Model file for the job. Use its own axes, mm. Face numbers are marked on the shaded views. A direction names the side the tool comes from. Coordinates: 2 decimals unless noted, no trailing zeros. Loops run counter-clockwise (first coordinate to the right, second up) from the corner with the lowest first, then second, coordinate; pieces in that order, holes last.
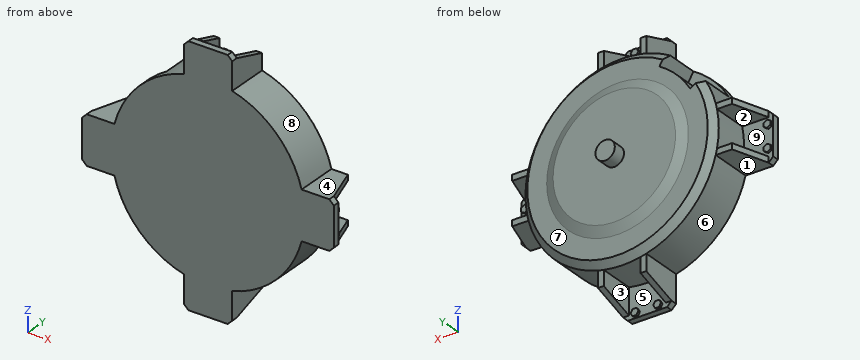
from build123d import *

# Parameters (mm, degrees)
SKETCH1_R                    = 150
BOSS_EXTRUDE1_DEPTH          = 75
CHAMFER1_SIZE                = 10
BOSS_EXTRUDE2_DEPTH          = 10
CHAMFER2_SIZE                = 7
BOSS_EXTRUDE3_DEPTH          = 9
BOSS_EXTRUDE4_DEPTH          = 3.5
CIRPATTERN1_COUNT            = 4
CIRPATTERN1_COPY_1_DEPTH     = 9
CIRPATTERN1_COPY_2_DEPTH     = 9
CIRPATTERN1_COPY_3_DEPTH     = 9
CIRPATTERN1_COPY_4_DEPTH     = 3.5
CIRPATTERN1_COPY_5_DEPTH     = 3.5
CIRPATTERN1_COPY_6_DEPTH     = 3.5
CHAMFER2_OF_CIRPATTERN1_SIZE = 7
CUT_EXTRUDE1_START           = -60
CUT_EXTRUDE1_DEPTH           = 60
SKETCH7_R                    = 110
SKETCH8_R                    = 95
SKETCH9_R                    = 15
BOSS_EXTRUDE5_DEPTH          = 20


with BuildPart() as part:
    # Sketch1 → Boss-Extrude1 (new body)
    with BuildSketch(Plane(origin=(0, 0, 0), x_dir=(1, 0, 0), z_dir=(0, 1, 0))):
        with Locations(Location((0, 0, 0), (0, 0, 270))):
            Circle(SKETCH1_R)
    extrude(amount=BOSS_EXTRUDE1_DEPTH)

    # Chamfer1
    chamfer1_edges = [part.edges().sort_by_distance(p)[0] for p in [
        (0, 75, -150),
    ]]
    chamfer(chamfer1_edges, length=CHAMFER1_SIZE)

    # Sketch2 → Boss-Extrude2 (add)
    with BuildSketch(Plane(origin=(0, 0, 0), x_dir=(-1, 0, 0), z_dir=(0, -1, 0))):
        with BuildLine():
            Line((145.236875483, 37.5), (195.236875483, 37.5))
            Line((195.236875483, 37.5), (195.236875483, -37.5))
            Line((195.236875483, -37.5), (145.236875483, -37.5))
            ThreePointArc((145.236875483, -37.5), (150, 0), (145.236875483, 37.5))
        make_face()
    boss_extrude2 = extrude(amount=-BOSS_EXTRUDE2_DEPTH)

    # Chamfer2
    chamfer2_edges = [part.edges().sort_by_distance(p)[0] for p in [
        (-195.236875483, 5, -37.5),
        (-195.236875483, 5, 37.5),
    ]]
    chamfer(chamfer2_edges, length=CHAMFER2_SIZE)

    # Sketch3 → Boss-Extrude3 (add)
    with BuildSketch(Plane.XY.offset(37.5)):
        Polygon((-145.236875483, 10), (-145.236875483, 65), (-170.556875483, 65), (-188.236875483, 10), align=None)
    boss_extrude3 = extrude(amount=-BOSS_EXTRUDE3_DEPTH)

    # Sketch4 → Boss-Extrude4 (add)
    with BuildSketch(Plane(origin=(0, 10, 0), x_dir=(1, 0, 0), z_dir=(0, 1, 0))):
        Polygon((-188.236875483, -23.54), (-183.04072306, -20.54), (-183.04072306, -14.54), (-188.236875483, -11.54), (-193.433027905, -14.54), (-193.433027905, -20.54), align=None)
    boss_extrude4 = extrude(amount=BOSS_EXTRUDE4_DEPTH)

    # Mirror1: Boss-Extrude3, Boss-Extrude4 across plane
    add(boss_extrude3.mirror(Plane.XY))
    add(boss_extrude4.mirror(Plane.XY))

    # CirPattern1: Boss-Extrude2, Boss-Extrude3, Boss-Extrude4 ×4 about axis
    cirpattern1_axis = Axis((0, 0, 0), (0, 1, 0))
    add([boss_extrude2.rotate(cirpattern1_axis, i * 360 / CIRPATTERN1_COUNT) for i in range(1, CIRPATTERN1_COUNT)])
    add([boss_extrude3.rotate(cirpattern1_axis, i * 360 / CIRPATTERN1_COUNT) for i in range(1, CIRPATTERN1_COUNT)])
    add([boss_extrude4.rotate(cirpattern1_axis, i * 360 / CIRPATTERN1_COUNT) for i in range(1, CIRPATTERN1_COUNT)])

    # CirPattern1 copy 1 sketch → CirPattern1 copy 1 (add)
    with BuildSketch(Plane(origin=(-37.5, 0, 0), x_dir=(0, 0, -1), z_dir=(-1, 0, 0))):
        Polygon((-145.236875483, -10), (-145.236875483, -65), (-170.556875483, -65), (-188.236875483, -10), align=None)
    extrude(amount=-CIRPATTERN1_COPY_1_DEPTH)

    # CirPattern1 copy 2 sketch → CirPattern1 copy 2 (add)
    with BuildSketch(Plane(origin=(0, 0, 37.5), x_dir=(-1, 0, 0), z_dir=(0, 0, 1))):
        Polygon((-145.236875483, -10), (-145.236875483, -65), (-170.556875483, -65), (-188.236875483, -10), align=None)
    extrude(amount=-CIRPATTERN1_COPY_2_DEPTH)

    # CirPattern1 copy 3 sketch → CirPattern1 copy 3 (add)
    with BuildSketch(Plane(origin=(37.5, 0, 0), x_dir=(0, 0, 1), z_dir=(1, 0, 0))):
        Polygon((-145.236875483, -10), (-145.236875483, -65), (-170.556875483, -65), (-188.236875483, -10), align=None)
    extrude(amount=-CIRPATTERN1_COPY_3_DEPTH)

    # CirPattern1 copy 4 sketch → CirPattern1 copy 4 (add)
    with BuildSketch(Plane(origin=(0, 10, 0), x_dir=(0, 0, -1), z_dir=(0, 1, 0))):
        Polygon((-188.236875483, 23.54), (-183.04072306, 20.54), (-183.04072306, 14.54), (-188.236875483, 11.54), (-193.433027905, 14.54), (-193.433027905, 20.54), align=None)
    extrude(amount=CIRPATTERN1_COPY_4_DEPTH)

    # CirPattern1 copy 5 sketch → CirPattern1 copy 5 (add)
    with BuildSketch(Plane(origin=(0, 10, 0), x_dir=(-1, 0, 0), z_dir=(0, 1, 0))):
        Polygon((-188.236875483, 23.54), (-183.04072306, 20.54), (-183.04072306, 14.54), (-188.236875483, 11.54), (-193.433027905, 14.54), (-193.433027905, 20.54), align=None)
    extrude(amount=CIRPATTERN1_COPY_5_DEPTH)

    # CirPattern1 copy 6 sketch → CirPattern1 copy 6 (add)
    with BuildSketch(Plane.ZX.offset(10)):
        Polygon((-188.236875483, 23.54), (-183.04072306, 20.54), (-183.04072306, 14.54), (-188.236875483, 11.54), (-193.433027905, 14.54), (-193.433027905, 20.54), align=None)
    extrude(amount=CIRPATTERN1_COPY_6_DEPTH)

    # Chamfer2 of CirPattern1
    chamfer2_of_cirpattern1_edges = [part.edges().sort_by_distance(p)[0] for p in [
        (-37.5, 5, 195.236875483),
        (37.5, 5, 195.236875483),
        (195.236875483, 5, 37.5),
        (195.236875483, 5, -37.5),
        (37.5, 5, -195.236875483),
        (-37.5, 5, -195.236875483),
    ]]
    chamfer(chamfer2_of_cirpattern1_edges, length=CHAMFER2_OF_CIRPATTERN1_SIZE)

    # Sketch6 → Cut-Extrude1 (cut)
    with BuildSketch(Plane(origin=(0, 75, 0), x_dir=(1, 0, 0), z_dir=(0, 1, 0)).offset(CUT_EXTRUDE1_START)):
        with BuildLine():
            Line((-112.583302492, -65), (-129.903810568, -75))
            ThreePointArc((-129.903810568, -75), (-106.066017178, -106.066017178), (-75, -129.903810568))
            Line((-75, -129.903810568), (-65, -112.583302492))
            ThreePointArc((-65, -112.583302492), (-91.923881554, -91.923881554), (-112.583302492, -65))
        make_face()
    extrude(amount=CUT_EXTRUDE1_DEPTH, mode=Mode.SUBTRACT)

    # Sketch7 → Loft1 section 0
    with BuildSketch(Plane(origin=(0, 75, 0), x_dir=(1, 0, 0), z_dir=(0, 1, 0))):
        Circle(SKETCH7_R)
    # Sketch8 → Loft1 section 1
    with BuildSketch(Plane(origin=(0, 82, 0), x_dir=(1, 0, 0), z_dir=(0, 1, 0))):
        Circle(SKETCH8_R)
    loft()

    # Sketch9 → Boss-Extrude5 (add)
    with BuildSketch(Plane(origin=(0, 82, 0), x_dir=(1, 0, 0), z_dir=(0, 1, 0))):
        with Locations(Location((0, 0, 0), (0, 0, 270))):
            Circle(SKETCH9_R)
    extrude(amount=BOSS_EXTRUDE5_DEPTH)


solid = part.part
Q1. Flat gauge pins, fed straight in: P1, Ø10, axis at x = 117.5, y = 29, coming from the -Z side; P2, Ø12, axis at x = 94.5, y = 62, coming from the +Z side; P3, Ø1.5, axis at x = -12, z = 133.5, coming from the +Y side. Where does each tip first touch, or does it go through?
Answers:
P1: stops at z = -99.22
P2: stops at z = 121.11
P3: stops at y = 75
Q2. Slice it at A-A (x = -157). List the corners of the cut face in (y, z).
Answers:
outline: (0, -37.5) - (65, -37.5) - (65, -28.5) - (10, -28.5) - (10, 28.5) - (65, 28.5) - (65, 37.5) - (0, 37.5) - close
Q3. Drill centre lines: line 1 (X direction, y = 47, z = -172.5); line 2 (X direction, y = 6.5, z = 149). Where is each one in solid material? Low to high.
Answers:
line 1: x = -37.5 to -28.5, 28.5 to 37.5
line 2: x = -37.5 to 37.5
Q4. Which spindle directions (+Z, -Z, +X, -X, +Y, -Y) get a long thin tool onto all of the face, cutting with end or side? Do the marked faces 1, 2, 3, 4 and 5. Say none if no direction does.
Answers:
face 1: -Z, -X, +Y, -Y
face 2: -X, +Y
face 3: -Z, +Y
face 4: +Z, +X, +Y, -Y
face 5: +Y
Q5. Slice it at B-B (x = 0). List the corners of the cut face in (y, z).
Answers:
outline: (0, -195.24) - (10, -195.24) - (10, -150) - (65, -150) - (75, -140) - (75, -110) - (82, -95) - (82, -15) - (102, -15) - (102, 15) - (82, 15) - (82, 95) - (75, 110) - (75, 140) - (65, 150) - (10, 150) - (10, 195.24) - (0, 195.24) - close
Q6. Mould opens along Z. For the marked faces 6, 7, 8 and 9 say: +Z half, -Z half, draft (parallel to the pull), parting line (faces both ways), or undercut.
Answers:
face 6: -Z half
face 7: draft
face 8: +Z half
face 9: undercut
